```python
from build123d import *

# Parameters (mm, degrees)
SKETCH_1_R           = 21
EXTRUDE_1_DEPTH      = 110
SKETCH_2_W           = 8
SKETCH_2_H           = 8
EXTRUDE_2_DEPTH      = 0.1
EXTRUDE_2_DEPTH_BACK = 55
SKETCH_3_R           = 175
EXTRUDE_3_DEPTH      = 15
SKETCH_4_R           = 125
SKETCH_4_R_2         = 116
EXTRUDE_4_DEPTH      = 5
SKETCH_5_R           = 116
SKETCH_5_R_2         = 40
CUT_EXTRUDE_1_DEPTH  = 8
CHAMFER_1_SIZE       = 1
SKETCH_6_R           = 9.5
CUT_EXTRUDE_2_DEPTH  = 16
SKETCH_7_R           = 125
EXTRUDE_5_DEPTH      = 68
SKETCH_8_R           = 140
EXTRUDE_6_DEPTH      = 322
SKETCH_9_R           = 144
EXTRUDE_7_DEPTH      = 145
CHAMFER_2_SIZE       = 60
EXTRUDE_8_DEPTH      = 260
CUT_EXTRUDE_3_REACH  = 337
SKETCH_11_R          = 7.5
SKETCH_12_W          = 120
SKETCH_12_H          = 120
EXTRUDE_9_DEPTH      = 245
SKETCH_13_R          = 35
EXTRUDE_10_DEPTH     = 150
CHAMFER_3_SIZE       = 1
SKETCH_15_R          = 12
SKETCH_16_R          = 16
EXTRUDE_11_DEPTH     = 14
EXTRUDE_12_DEPTH     = 16
SKETCH_18_R          = 7
CUT_EXTRUDE_4_DEPTH  = 16


with BuildPart() as part:
    # Эскиз1 → Вытянуть1 (new body)
    with BuildSketch(Plane.XY):
        Circle(SKETCH_1_R)
    extrude(amount=EXTRUDE_1_DEPTH)

    # Эскиз2 → Вытянуть2 (add, two sides)
    with BuildSketch(Plane(origin=(0, 0, 0), x_dir=(-1, 0, 0), z_dir=(0, 0, -1))) as extrude_2_sk:
        with Locations((0, 20)):
            Rectangle(SKETCH_2_W, SKETCH_2_H)
    extrude(amount=EXTRUDE_2_DEPTH)
    extrude(extrude_2_sk.sketch, amount=-EXTRUDE_2_DEPTH_BACK)

    # Эскиз3 → Вытянуть3 (add)
    with BuildSketch(Plane.XY.offset(110)):
        Circle(SKETCH_3_R)
    extrude(amount=EXTRUDE_3_DEPTH)

    # Эскиз4 → Вытянуть4 (add)
    with BuildSketch(Plane(origin=(0, 0, 110), x_dir=(-1, 0, 0), z_dir=(0, 0, -1))):
        with Locations(Location((0, 0, 0), (0, 0, 180))):  # turned: the seam where the file's is
            Circle(SKETCH_4_R)
        Circle(SKETCH_4_R_2, mode=Mode.SUBTRACT)
    extrude(amount=EXTRUDE_4_DEPTH)

    # Эскиз5 → Вырез-Вытянуть1 (cut)
    with BuildSketch(Plane(origin=(0, 0, 110), x_dir=(-1, 0, 0), z_dir=(0, 0, -1))):
        Circle(SKETCH_5_R)
        Circle(SKETCH_5_R_2, mode=Mode.SUBTRACT)
    extrude(amount=-CUT_EXTRUDE_1_DEPTH, mode=Mode.SUBTRACT)

    # Фаска1
    chamfer_1_edges = [part.edges().sort_by_distance(p)[0] for p in [
        (-125, 0, 105),
        (40, 0, 110),
        (-13.360389216, -16.201851746, 0),
    ]]
    chamfer(chamfer_1_edges, length=CHAMFER_1_SIZE)

    # Эскиз6 → Вырез-Вытянуть2 (cut, through all)
    with BuildSketch(Plane(origin=(0, 0, 110), x_dir=(-1, 0, 0), z_dir=(0, 0, -1))):
        with Locations((-57.402514855, 138.581929877)):
            Circle(SKETCH_6_R)
        with Locations((57.402514855, 138.581929877)):
            Circle(SKETCH_6_R)
        with Locations((138.581929877, 57.402514855)):
            Circle(SKETCH_6_R)
        with Locations((138.581929877, -57.402514855)):
            Circle(SKETCH_6_R)
        with Locations((57.402514855, -138.581929877)):
            Circle(SKETCH_6_R)
        with Locations((-57.402514855, -138.581929877)):
            Circle(SKETCH_6_R)
        with Locations((-138.581929877, -57.402514855)):
            Circle(SKETCH_6_R)
        with Locations((-138.581929877, 57.402514855)):
            Circle(SKETCH_6_R)
    extrude(amount=-CUT_EXTRUDE_2_DEPTH, mode=Mode.SUBTRACT)

    # Эскиз7 → Вытянуть5 (add)
    with BuildSketch(Plane.XY.offset(125)):
        Circle(SKETCH_7_R)
    extrude(amount=EXTRUDE_5_DEPTH)

    # Эскиз8 → Вытянуть6 (add)
    with BuildSketch(Plane.XY.offset(193)):
        Circle(SKETCH_8_R)
    extrude(amount=EXTRUDE_6_DEPTH)

    # Эскиз9 → Вытянуть7 (add)
    with BuildSketch(Plane.XY.offset(515)):
        Circle(SKETCH_9_R)
    extrude(amount=EXTRUDE_7_DEPTH)

    # Фаска2
    chamfer_2_edges = [part.edges().sort_by_distance(p)[0] for p in [
        (-144, 0, 660),
    ]]
    chamfer(chamfer_2_edges, length=CHAMFER_2_SIZE)

    # Эскиз10 → Вытянуть8 (add)
    with BuildSketch(Plane(origin=(0, 0, 193), x_dir=(-1, 0, 0), z_dir=(0, 0, -1))):
        Polygon((-152, -160), (-91.607695155, -160), (-51.945448858, -91.302974272), (-67.533906126, -82.302974272), (-102, -142), (-152, -142), align=None)
        Polygon((91.607695155, -160), (51.945448858, -91.302974272), (67.533906126, -82.302974272), (102, -142), (152, -142), (152, -160), align=None)
    extrude(amount=-EXTRUDE_8_DEPTH)

    # Эскиз11 → Вырез-Вытянуть3 (cut, up to next)
    with BuildSketch(Plane.XZ.offset(160), mode=Mode.PRIVATE) as cut_extrude_3_sk1:
        with Locations((-127, 218)):
            Circle(SKETCH_11_R)
    cut_extrude_3_tool1 = extrude(cut_extrude_3_sk1.sketch, amount=-CUT_EXTRUDE_3_REACH, mode=Mode.PRIVATE) & part.part
    add(cut_extrude_3_tool1.solids().sort_by_distance((-127, -160, 218))[0], mode=Mode.SUBTRACT)
    # Эскиз11 → Вырез-Вытянуть3 (cut, up to next)
    with BuildSketch(Plane.XZ.offset(160), mode=Mode.PRIVATE) as cut_extrude_3_sk2:
        with Locations((127, 218)):
            Circle(SKETCH_11_R)
    cut_extrude_3_tool2 = extrude(cut_extrude_3_sk2.sketch, amount=-CUT_EXTRUDE_3_REACH, mode=Mode.PRIVATE) & part.part
    add(cut_extrude_3_tool2.solids().sort_by_distance((127, -160, 218))[0], mode=Mode.SUBTRACT)
    # Эскиз11 → Вырез-Вытянуть3 (cut, up to next)
    with BuildSketch(Plane.XZ.offset(160), mode=Mode.PRIVATE) as cut_extrude_3_sk3:
        with Locations((-127, 428)):
            Circle(SKETCH_11_R)
    cut_extrude_3_tool3 = extrude(cut_extrude_3_sk3.sketch, amount=-CUT_EXTRUDE_3_REACH, mode=Mode.PRIVATE) & part.part
    add(cut_extrude_3_tool3.solids().sort_by_distance((-127, -160, 428))[0], mode=Mode.SUBTRACT)
    # Эскиз11 → Вырез-Вытянуть3 (cut, up to next)
    with BuildSketch(Plane.XZ.offset(160), mode=Mode.PRIVATE) as cut_extrude_3_sk4:
        with Locations((127, 428)):
            Circle(SKETCH_11_R)
    cut_extrude_3_tool4 = extrude(cut_extrude_3_sk4.sketch, amount=-CUT_EXTRUDE_3_REACH, mode=Mode.PRIVATE) & part.part
    add(cut_extrude_3_tool4.solids().sort_by_distance((127, -160, 428))[0], mode=Mode.SUBTRACT)

    # Эскиз12 → Вытянуть9 (add)
    with BuildSketch(Plane(origin=(0, 0, 0), x_dir=(1, 0, 0), z_dir=(0, 1, 0))):
        with Locations((0, -254)):
            Rectangle(SKETCH_12_W, SKETCH_12_H)
    extrude(amount=EXTRUDE_9_DEPTH)

    # Эскиз13 → Вытянуть10 (add)
    with BuildSketch(Plane(origin=(0, 0, 0), x_dir=(1, 0, 0), z_dir=(0, 1, 0))):
        with Locations(Location((0, -371, 0), (0, 0, 90))):  # turned: the seam where the file's is
            Circle(SKETCH_13_R)
    extrude(amount=EXTRUDE_10_DEPTH)

    # Фаска3
    chamfer_3_edges = [part.edges().sort_by_distance(p)[0] for p in [
        (0, 150, 406),
    ]]
    chamfer(chamfer_3_edges, length=CHAMFER_3_SIZE)

    # По траектории1: sweep along a path in Эскиз14
    with BuildLine(Plane.XY.offset(370)) as sweep_1_path:
        CenterArc((0, 188), 38, 0, 360)
    # Эскиз15 → По траектории1 (sweep)
    with BuildSketch(Plane(origin=(0, 0, 0), x_dir=(0, 0, -1), z_dir=(1, 0, 0))):
        with Locations((-370, 226)):
            Circle(SKETCH_15_R)
    sweep(path=sweep_1_path.line)

    # Эскиз16 → Вытянуть11 (add)
    with BuildSketch(Plane.ZY.offset(60)):
        with Locations(Location((254, 185, 0), (0, 0, 180))):  # turned: the seam where the file's is
            Circle(SKETCH_16_R)
    extrude(amount=EXTRUDE_11_DEPTH)

    # Эскиз17 → Вытянуть12 (add)
    with BuildSketch(Plane.ZY.offset(74)):
        Polygon((254, 207.516660498), (234.5, 196.258330249), (234.5, 173.741669751), (254, 162.483339502), (273.5, 173.741669751), (273.5, 196.258330249), align=None)
    extrude(amount=EXTRUDE_12_DEPTH)

    # Эскиз18 → Вырез-Вытянуть4 (cut)
    with BuildSketch(Plane.ZY.offset(90)):
        with Locations((254, 185)):
            Circle(SKETCH_18_R)
    extrude(amount=-CUT_EXTRUDE_4_DEPTH, mode=Mode.SUBTRACT)


solid = part.part
```
Design review of the part built by this model. Coordinates are the model's own, in mm. A direction names the side the tool comes from. Round coordinates to 2 decimals unless told otherwise and drop trailing zeros. Write each loop counter-clockwise with the first axis right and the second up, starting at its lowest first coordinate (ties: lowest second). Pieces come first, ordered by that corner, then holes. Notation, with made-up numbers: (44.5, 58.5) -> (54.5, 58.5) arc R19 cw to (54.5, 80.5) -> close; hole circle Ø6 at (-26.75, -2). An arc over 180 degrees is marked (long way). Write item = value, one per line. Start each with the question number.
1) Take a section at A-A, the plane z = 218. State the section outline as (x, y) points, plus the area to 3 significant figures.
2) Tool access review of faces 1 (the face through (8.67, -39.05, 114.45)), 2 (the face through (-81.9, 168.2, 244.1)), 3 (the face through (-18.841, -84.847, 657.087)), 4 (the face through (-66.9, 180.19, 238.74)): name each direction out of +Z, -Z, +X, -X, +Y, -Y from which nothing blocks a thin tool from reaching the whole face with its end or side.
3) Mouldability with a two-part tool opening along X and no side actions: class faces 5 (the face through (146.121, -63.183, 117.395)), 6 (the face through (-93.114, -126.609, 321.18)), 7 (the face through (122, -160, 321)) as +X half, -X half, draft (parallel to the pull), parting line (faces both ways), or undercut.
4) Take a section at C-C, the plane z = 70. State the section outline as (x, y) points.
5) Take a section at B-B, the plane z = 428. State the section outline as (x, y) points.
6) Clearance check with flat-ended pins moving along their axes: pin 1 (10 mm diameter, centred on x = 85.5, z = 195, fed in from -Y); pin 2 (15 mm diameter, centred on x = 138.58, y = -57.4, fed in from +Z); pin 3 (3 mm diameter, centred on x = 123, y = 31, fed in from +Z). State where each tip first meets the part, or that it passes through.
7) Wall thickness on probe 1 along Y at (x, z) = (-78, 254); probe 2 along X at (y, z) = (-149, 428); probe 3 along Y at (x, z) = (147, 205.5): over which ranges is each line inside the solid? List them lowest first. Write a range as from..to.
Results list:
q1.outline = (-152, -160) -> (-134.5, -160) -> (-134.5, -142) -> (-152, -142) -> close; (-119.5, -160) -> (-91.61, -160) -> (-69.42, -121.57) arc R140 ccw to (69.42, -121.57) -> (91.61, -160) -> (119.5, -160) -> (119.5, -142) -> (102, -142) -> (84.47, -111.64) arc R140 ccw to (60, 126.49) -> (60, 245) -> (-60, 245) -> (-60, 126.49) arc R140 ccw to (-84.47, -111.64) -> (-102, -142) -> (-119.5, -142) -> close; (134.5, -160) -> (152, -160) -> (152, -142) -> (134.5, -142) -> close
q1.area = 77,600 mm²
q2.face_1 = -Z
q2.face_2 = -Z, -X
q2.face_3 = +Z
q2.face_4 = none
q3.face_5 = undercut
q3.face_6 = -X half
q3.face_7 = draft
q4.outline = circle Ø42 at (0, 0)
q5.outline = (-152, -160) -> (-134.5, -160) -> (-134.5, -142) -> (-152, -142) -> close; (-119.5, -160) -> (-91.61, -160) -> (-69.42, -121.57) arc R140 ccw to (69.42, -121.57) -> (91.61, -160) -> (119.5, -160) -> (119.5, -142) -> (102, -142) -> (84.47, -111.64) arc R140 ccw (long way) to (-84.47, -111.64) -> (-102, -142) -> (-119.5, -142) -> close; (134.5, -160) -> (152, -160) -> (152, -142) -> (134.5, -142) -> close
q6.pin_1 = -158.08
q6.pin_2 = 601.5
q6.pin_3 = 618.65
q7.probe_1 = -136.43..116.26, 162.48..178, 192..207.52
q7.probe_2 = -152..-134.5, -119.5..-85.26, 85.26..119.5, 134.5..152
q7.probe_3 = -160..-142
